Check sheet for the modelled part. Datum: model origin and axes. Units: mm. Round coordinates to 2 decimals unless told otherwise and drop trailing zeros. Order: outer loops, then holes, each group sorted by start corner. A loop starts at its lowest first (then second) coordinate and runs counter-clockwise, first axis right, second up.
from build123d import *

# Parameters (mm, degrees)
SKETCH_1_R                = 33.5
EXTRUDE_1_DEPTH           = 4
SKETCH_2_R                = 2.15
CUT_EXTRUDE_1_DEPTH       = 24
SKETCH_3_R                = 4.5
CUT_EXTRUDE_2_DEPTH       = 5
SKETCH_4_R                = 11.2
CUT_EXTRUDE_3_DEPTH       = 5
HOLE_WIZARD_1_D           = 3.3
HOLE_WIZARD_1_CSINK_D     = 6
HOLE_WIZARD_1_CSINK_ANGLE = 90
SKETCH_9_R                = 2.15
SKETCH_9_R_2              = 4.5
SKETCH_9_R_3              = 3
EXTRUDE_2_DEPTH           = 4
SKETCH_10_R               = 2.15
CUT_EXTRUDE_4_DEPTH       = 4
FILLET_1_R                = 3


with BuildPart() as part:
    # 草图1 → 凸台-拉伸1 (new body)
    with BuildSketch(Plane(origin=(0, 0, 0), x_dir=(1, 0, 0), z_dir=(0, 1, 0))):
        Circle(SKETCH_1_R)
    extrude(amount=EXTRUDE_1_DEPTH)

    # 草图2 → 切除-拉伸1 (cut)
    with BuildSketch(Plane(origin=(0, 4, 0), x_dir=(1, 0, 0), z_dir=(0, 1, 0))):
        with Locations((-18.950679053, 21.951577698)):
            Circle(SKETCH_2_R)
        with Locations((9.535284413, 27.387558328)):
            Circle(SKETCH_2_R)
        with Locations((28.485963466, 5.43598063)):
            Circle(SKETCH_2_R)
        with Locations((18.950679053, -21.951577698)):
            Circle(SKETCH_2_R)
        with Locations((-9.535284413, -27.387558328)):
            Circle(SKETCH_2_R)
        with Locations((-28.485963466, -5.43598063)):
            Circle(SKETCH_2_R)
    extrude(amount=-CUT_EXTRUDE_1_DEPTH, mode=Mode.SUBTRACT)

    # 草图3 → 切除-拉伸2 (cut, through all)
    with BuildSketch(Plane(origin=(0, 4, 0), x_dir=(1, 0, 0), z_dir=(0, 1, 0))):
        with Locations((-18.172080142, -3.467780747)):
            Circle(SKETCH_3_R)
        with Locations((-6.329456033, -18.179672338)):
            Circle(SKETCH_3_R)
    extrude(amount=-CUT_EXTRUDE_2_DEPTH, mode=Mode.SUBTRACT)

    # 草图4 → 切除-拉伸3 (cut, through all)
    with BuildSketch(Plane(origin=(0, 4, 0), x_dir=(1, 0, 0), z_dir=(0, 1, 0))):
        Circle(SKETCH_4_R)
    extrude(amount=-CUT_EXTRUDE_3_DEPTH, mode=Mode.SUBTRACT)

    # 孔1 (through all)
    with Locations(Plane(origin=(12.774024908, 0, -9.317955122), x_dir=(0, 0, -1), z_dir=(0, -1, 0))):
        with Locations((0, 0), (4.110036385, -11.804982038), (-24.554362639, -8.548875681), (-20.444326254, -20.353857719)):
            CounterSinkHole(HOLE_WIZARD_1_D / 2, HOLE_WIZARD_1_CSINK_D / 2, counter_sink_angle=HOLE_WIZARD_1_CSINK_ANGLE)

    # 草图9 → 凸台-拉伸2 (add)
    with BuildSketch(Plane.XZ):
        with BuildLine():
            ThreePointArc((30.94197409, -12.839168175), (11.014897512, -31.637351862), (-16.277954062, -29.279313714))
            Line((-16.277954062, -29.279313714), (-5.854606893, -59.217595173))
            Line((-5.854606893, -59.217595173), (41.365321259, -42.777449634))
            Line((41.365321259, -42.777449634), (30.94197409, -12.839168175))
        make_face()
        with BuildLine():
            Line((-19.548240775, -19.886288375), (-23.609964076, -8.22007277))
            Line((-23.609964076, -8.22007277), (-10.577263906, -3.682592601))
            ThreePointArc((-10.577263906, -3.682592601), (-10.882752845, 2.646826497), (-7.704540242, 8.128964243))
            ThreePointArc((-7.704540242, 8.128964243), (-10.570999096, 10.896318406), (-8.161427671, 14.069455809))
            ThreePointArc((-8.161427671, 14.069455809), (-5.543963925, 22.610586708), (-6.021999809, 13.690187884))
            ThreePointArc((-6.021999809, 13.690187884), (-4.757437603, 12.143270974), (-4.744786266, 10.145294638))
            ThreePointArc((-4.744786266, 10.145294638), (4.352709301, 10.319589223), (10.577263906, 3.682592601))
            Line((10.577263906, 3.682592601), (23.609964076, 8.22007277))
            Line((23.609964076, 8.22007277), (27.671687377, -3.446142835))
            ThreePointArc((27.671687377, -3.446142835), (29.684255252, -3.650876488), (30.635963466, -5.43598063))
            ThreePointArc((30.635963466, -5.43598063), (30.204575944, -6.727828589), (29.083525188, -7.501269953))
            Line((29.083525188, -7.501269953), (30.94197409, -12.839168175))
            ThreePointArc((30.94197409, -12.839168175), (32.854270134, -6.545756946), (33.5, 0))
            ThreePointArc((33.5, 0), (-16.984383105, 28.875261566), (-16.277954062, -29.279313714))
            Line((-16.277954062, -29.279313714), (-18.136402964, -23.941415493))
            ThreePointArc((-18.136402964, -23.941415493), (-20.981135964, -22.658503956), (-19.548240775, -19.886288375))
        make_face()
        with Locations((-28.485963466, 5.43598063)):
            Circle(SKETCH_9_R, mode=Mode.SUBTRACT)
        with Locations((-18.172080142, 3.467780747)):
            Circle(SKETCH_9_R_2, mode=Mode.SUBTRACT)
        with Locations((-9.535284413, 27.387558328)):
            Circle(SKETCH_9_R, mode=Mode.SUBTRACT)
        with Locations((4.225149227, 15.236407517)):
            Circle(SKETCH_9_R_3, mode=Mode.SUBTRACT)
        with Locations((18.950679053, 21.951577698)):
            Circle(SKETCH_9_R, mode=Mode.SUBTRACT)
    extrude(amount=-EXTRUDE_2_DEPTH)

    # 草图10 → 切除-拉伸4 (cut)
    with BuildSketch(Plane.XZ):
        with Locations((16.356125201, -40.895930952)):
            Circle(SKETCH_10_R)
        with Locations((23.911313705, -38.265507665)):
            Circle(SKETCH_10_R)
    extrude(amount=-CUT_EXTRUDE_4_DEPTH, mode=Mode.SUBTRACT)

    # 圆角1
    fillet_1_edges = [part.edges().sort_by_distance(p)[0] for p in [
        (30.94197409, 2, -12.839168175),
        (-16.277954062, 2, -29.279313714),
        (-5.854606893, 2, -59.217595173),
        (41.365321259, 2, -42.777449634),
    ]]
    fillet(fillet_1_edges, radius=FILLET_1_R)


solid = part.part
1) Gauge pin test, flat ends, axial feed: pin 1 (4 mm diameter, centred on x = 23.91, z = -38.27, fed in from +Y); pin 2 (1.5 mm diameter, centred on y = 1, z = 16, fed in from -X); pin 3 (2 mm diameter, centred on x = 11.5, y = 2.5, fed in from +Z). Record the tip position at first contact, or that the pin passes through.
2) Sectioned sample at B-B on z = -34. Record the cut outline in (x, y).
3) Draft check along Z on faces 1 (the face through (-11.44, 1.97, -43.18)), 2 (the face through (40.23, 2.03, -42.27)), 3 (the face through (23.445, 1.972, -40.364)). Enter one of: pulls with the +Z half, pulls with the -Z half, needs draft (parallel to the pull), parting line crosses it, or undercut.
4) Scan lines: line 1 (Z direction, x = -1, y = 0.7); line 2 (Z direction, x = 5, y = 0.3); line 3 (X direction, y = 2.4, z = 0). Record each from-to range of solid material in increasing order.
5) Sectioned sample at A-A on z = 0. Record the cut outline in (x, y).
6) Sectioned sample at C-C on z = -47.5. Record the cut outline in (x, y).
Values found:
1. pin 1: passes through
1. pin 2: stops at x = -29.83
1. pin 3: stops at z = 31.81
2. outline: (-14.63, 0) - (38.31, 0) - (38.31, 4) - (-14.63, 4) - close
3. face 1: pulls with the -Z half
3. face 2: parting line crosses it
3. face 3: undercut
4. line 1: z = -57.53 to -14.62, -12.24 to -11.16, 11.16 to 33.49
4. line 2: z = -55.44 to -10.02, 10.02 to 12.65, 17.82 to 33.12
4. line 3: x = -33.5 to -21.04, -15.3 to -11.2, 11.2 to 33.5
5. outline: (-33.5, 0) - (-21.04, 0) - (-21.04, 4) - (-33.5, 4) - close; (-15.3, 0) - (-11.2, 0) - (-11.2, 4) - (-15.3, 4) - close; (11.2, 0) - (33.5, 0) - (33.5, 4) - (11.2, 4) - close
6. outline: (-9.93, 0) - (27.8, 0) - (27.8, 4) - (-9.93, 4) - close
